Geometry: final body of the model. Coordinates: model frame, mm. Give positions to 0.01 mm unless a question says otherwise; leave off trailing zeros. Order: outer loops, then holes, each group sorted by start corner. A loop starts at its lowest first (then second) coordinate and runs counter-clockwise, first axis right, second up. Notation, with made-up numbers: (19, 79) - (48, 79) arc R12 cw to (48, 96) - close; hole circle Ø6 at (7, -15). An arc over 180 degrees is marked (long way). Use one line per item in the form item = value.
from build123d import *

# Parameters (mm, degrees)
SKETCH1_R           = 2.65
SKETCH1_R_2         = 2.55
SKETCH1_R_3         = 4.5
SKETCH1_W           = 25
SKETCH1_H           = 5
BOSS_EXTRUDE1_DEPTH = 5


with BuildPart() as part:
    # Sketch1 → Boss-Extrude1 (new body)
    with BuildSketch(Plane(origin=(0, 0, 0), x_dir=(1, 0, 0), z_dir=(0, 1, 0))):
        Polygon((0, 0), (0, 40), (0, 65), (-336.537, 65), (-336.537, 38.5), (-368.537, 38.5), (-368.537, -65), (0, -65), align=None)
        with Locations(Location((-12, 42.5, 0), (0, 0, 270))):
            Circle(SKETCH1_R, mode=Mode.SUBTRACT)
        with Locations(Location((-24.537, 33.50840474, 0), (0, 0, 270))):
            Circle(SKETCH1_R_2, mode=Mode.SUBTRACT)
        with Locations(Location((-24.537, -2.49159526, 0), (0, 0, 270))):
            Circle(SKETCH1_R_2, mode=Mode.SUBTRACT)
        with Locations(Location((-24.537, 15.50840474, 0), (0, 0, 270))):
            Circle(SKETCH1_R_3, mode=Mode.SUBTRACT)
        with Locations(Location((-12, -11.5, 0), (0, 0, 270))):
            Circle(SKETCH1_R, mode=Mode.SUBTRACT)
        with Locations(Location((-334.037, -51, 0), (0, 0, 270))):
            Circle(SKETCH1_R, mode=Mode.SUBTRACT)
        with Locations(Location((-234.037, -51, 0), (0, 0, 270))):
            Circle(SKETCH1_R, mode=Mode.SUBTRACT)
        with Locations(Location((-134.037, -51, 0), (0, 0, 270))):
            Circle(SKETCH1_R, mode=Mode.SUBTRACT)
        with Locations(Location((-34.037, -51, 0), (0, 0, 270))):
            Circle(SKETCH1_R, mode=Mode.SUBTRACT)
        with Locations(Location((-52, -11.5, 0), (0, 0, 270))):
            Circle(SKETCH1_R, mode=Mode.SUBTRACT)
        with Locations(Location((-52, 42.5, 0), (0, 0, 270))):
            Circle(SKETCH1_R, mode=Mode.SUBTRACT)
        with BuildLine():
            Line((-358.537, 20), (-344.537, 20))
            ThreePointArc((-344.537, 20), (-340.037, 15.5), (-344.537, 11))
            Line((-344.537, 11), (-358.537, 11))
            ThreePointArc((-358.537, 11), (-363.037, 15.5), (-358.537, 20))
        make_face(mode=Mode.SUBTRACT)
        with BuildLine():
            Line((-344.5, 0.05), (-358.5, 0.05))
            ThreePointArc((-358.5, 0.05), (-361.05, -2.5), (-358.5, -5.05))
            Line((-358.5, -5.05), (-344.5, -5.05))
            ThreePointArc((-344.5, -5.05), (-341.95, -2.5), (-344.5, 0.05))
        make_face(mode=Mode.SUBTRACT)
        with Locations((-122.055571099, 37)):
            Rectangle(SKETCH1_W, SKETCH1_H, mode=Mode.SUBTRACT)
        with BuildLine():
            Line((-358.5, 36.05), (-344.5, 36.05))
            ThreePointArc((-344.5, 36.05), (-341.95, 33.5), (-344.5, 30.95))
            Line((-344.5, 30.95), (-358.5, 30.95))
            ThreePointArc((-358.5, 30.95), (-361.05, 33.5), (-358.5, 36.05))
        make_face(mode=Mode.SUBTRACT)
        with Locations((-72.055571099, 37)):
            Rectangle(SKETCH1_W, SKETCH1_H, mode=Mode.SUBTRACT)
        with Locations((-272.055571099, 37)):
            Rectangle(SKETCH1_W, SKETCH1_H, mode=Mode.SUBTRACT)
        with Locations((-222.055571099, 37)):
            Rectangle(SKETCH1_W, SKETCH1_H, mode=Mode.SUBTRACT)
        with Locations((-172.055571099, 37)):
            Rectangle(SKETCH1_W, SKETCH1_H, mode=Mode.SUBTRACT)
    extrude(amount=BOSS_EXTRUDE1_DEPTH)


solid = part.part
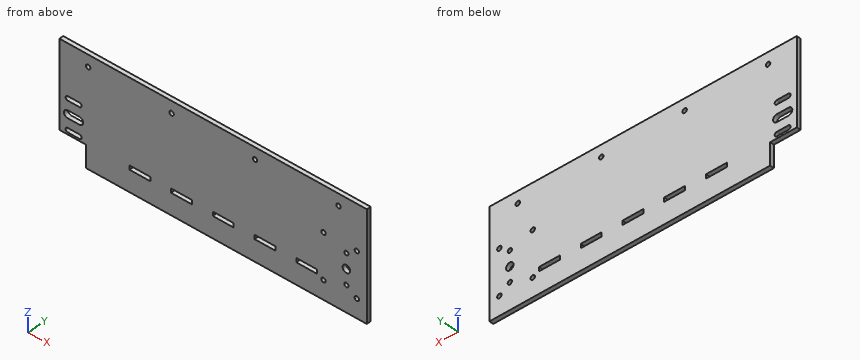
(1) Ray query, line 1 along X through (y, z) = (2.1, 51); line 2 along X through (y, z) = (1.75, -33.5); line 3 along Z through (x, y) = (-73, 4.8). Return the intervals inside material, ascending.
Computed values:
line_1 = -368.54 to -336.69, -331.39 to -236.69, -231.39 to -136.69, -131.39 to -36.69, -31.39 to 0
line_2 = -368.54 to -361.05, -341.95 to -27.09, -21.99 to 0
line_3 = -65 to -39.5, -34.5 to 65
(2) Contact query for flat-ended pins moving along their axis: pin 1 Ø5 at (x, z) = (-34.037, 51) entering from -Y; pin 2 Ø2.5 at (x, y) = (-348.5, 1.5) entering from -Z. Output: stop coordinate, or through.
Computed values:
pin_1 = through
pin_2 = -38.5
(3) Cut plane B-B on x = -79. Output: boundary loops of the cut face in (y, z), plus the area to 3 significant figures.
Computed values:
outline = (0, -65) - (5, -65) - (5, -39.5) - (0, -39.5) - close; (0, -34.5) - (5, -34.5) - (5, 65) - (0, 65) - close
area = 625 mm²
(4) Cut plane A-A on z = -15.5. Output: boundary loops of the cut face in (x, y), plus the area to 3 significant figures.
Computed values:
outline = (-368.54, 0) - (-363.04, 0) - (-363.04, 5) - (-368.54, 5) - close; (-340.04, 0) - (-29.04, 0) - (-29.04, 5) - (-340.04, 5) - close; (-20.04, 0) - (0, 0) - (0, 5) - (-20.04, 5) - close
area = 1,680 mm²
(5) Cut plane C-C on z = -53. Output: boundary loops of the cut face in (x, y).
Computed values:
outline = (-336.54, 0) - (0, 0) - (0, 5) - (-336.54, 5) - close
(6) Cut plane D-D on y = 1.85. Give the number of separate pieces and of enclosed holes in the cut face, plus the area to 3 significant figures.
Computed values:
separate_pieces = 1
enclosed_holes = 19
area = 45,800 mm²
